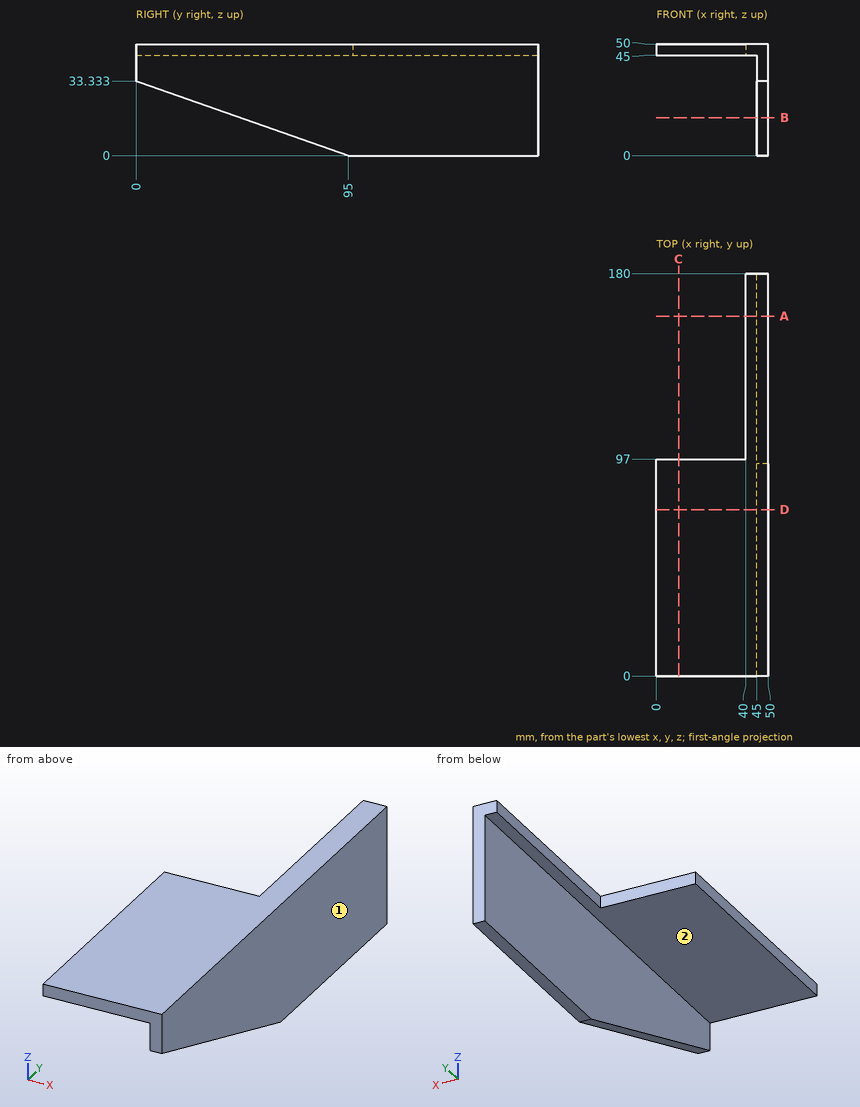
The figure shows three views and two pictorial views of one solid part (mm, origin at its lowest corner). Answer the questions. A direction names the side the tool comes from. Round coordinates to 2 decimals unless told otherwise and drop trailing zeros. Loops run counter-clockwise (first coordinate to the right, second up) from the corner with the lowest first, then second, coordinate; pieces in that order, holes last. Notation, with made-up numbers: M 11.5,73 L 17.5,73 A16 cw 17.5,88 Z; hole C 42,84.25 d11. An arc over 180 degrees is marked long. Return JSON: item names as keys, results as strings.
Q1. Find section D-D, the plane y = 74.5. Determine the outline of the cut face in (x, z), plus the area to 3 significant figures.
Results list:
{"outline": "M 0,45 L 45,45 L 45,7.19 L 50,7.19 L 50,50 L 0,50 Z", "area": "439 mm2"}
Q2. Find section C-C, the plane x = 10. Determine the outline of the cut face in (y, z), plus the area to 3 significant figures.
Results list:
{"outline": "M 0,45 L 97,45 L 97,50 L 0,50 Z", "area": "485 mm2"}
Q3. Find the intervals of material crossed by line 1 along Z through (x, y) = (24, 84.5), in increasing order. Write a range as from..to.
Results list:
{"line 1": "z = 45..50"}
Q4. Find section B-B, the plane z = 17. Determine the outline of the cut face in (x, y), plus the area to 3 significant figures.
Results list:
{"outline": "M 45,46.55 L 50,46.55 L 50,180 L 45,180 Z", "area": "667 mm2"}
Q5. Find section A-A, the plane y = 161. Determine the outline of the cut face in (x, z).
Results list:
{"outline": "M 40,45 L 45,45 L 45,0 L 50,0 L 50,50 L 40,50 Z"}
Q6. Each of these flat-tipped pins is pushed along its axis until it touches: pin 1 Ø8 at (y, z) = (96.5, 30.5) entering from -X; pin 2 Ø2.5 at (x, z) = (14, 48) entering from +Y; pin 3 Ø22.5 at (x, y) = (26.5, 64) entering from -Z. Where does it stop, or does it pass through?
Results list:
{"pin 1": "stops at x = 45", "pin 2": "stops at y = 97", "pin 3": "stops at z = 45"}
Q7. Which of the six approach directions +Z, -Z, +X, -X, +Y, -Y give full straight-line access (tool end or side, diameter ignored) to the marked faces 1 and 2?
Results list:
{"face 1": "+Z, -Z, +X, +Y, -Y", "face 2": "-Z, -X, +Y, -Y"}
